```python
from build123d import *

# Parameters (mm, degrees)
CYLINDER014_R     = 1.2
CYLINDER014_DEPTH = 3
CYLINDER013_R     = 0.5
CYLINDER013_DEPTH = 10
ARRAY013_X_COUNT  = 2
ARRAY013_X_PITCH  = 8
ARRAY013_Y_COUNT  = 2
ARRAY013_Y_PITCH  = 8
BOX016_W          = 8
BOX016_H          = 8
BOX016_DEPTH      = 10
TORUS_R           = 0.7
CYLINDER012_R     = 7.7
CYLINDER012_DEPTH = 2.4
CYLINDER003_R     = 10
CYLINDER003_DEPTH = 1.4


with BuildPart() as magnet:
    # Cylinder014 → Cylinder014 (new body)
    with BuildSketch(Plane(origin=(0, -8.5, -1), x_dir=(1, 0, 0), z_dir=(0, 0, 1))):
        Circle(CYLINDER014_R)
    extrude(amount=CYLINDER014_DEPTH)


with BuildPart() as array013:
    # Cylinder013 → Cylinder013 (new body)
    with BuildSketch(Plane(origin=(4, 4, -2), x_dir=(1, 0, 0), z_dir=(0, 0, 1))):
        Circle(CYLINDER013_R)
    extrude(amount=CYLINDER013_DEPTH)

    # Array013 X: Array013 ×2


with BuildPart() as array013_1:
    add(array013.part)
    with Locations(*[(-i * ARRAY013_X_PITCH, 0, 0) for i in range(1, ARRAY013_X_COUNT)]):
        add(array013.part)

    # Array013 Y: Array013 ×2


with BuildPart() as array013_2:
    add(array013_1.part)
    with Locations(*[(0, -i * ARRAY013_Y_PITCH, 0) for i in range(1, ARRAY013_Y_COUNT)]):
        add(array013_1.part)


with BuildPart() as obj1:
    # Box016 → Box016 (new body)
    with BuildSketch(Plane(origin=(-4, -4, -2), x_dir=(1, 0, 0), z_dir=(0, 0, 1))):
        with Locations((4, 4)):
            Rectangle(BOX016_W, BOX016_H)
    extrude(amount=BOX016_DEPTH)


with BuildPart() as torus:
    # Torus → Torus (revolve)
    with BuildSketch(Plane(origin=(0, 0, 1.9), x_dir=(1, 0, 0), z_dir=(0, -1, 0))):
        with Locations((7.7, 0)):
            Circle(TORUS_R)
    revolve(axis=Axis((0, 0, 1.9), (0, 0, 1)))


with BuildPart() as cut017:
    # Cylinder012 → Cylinder012 (new body)
    with BuildSketch(Plane.XY):
        Circle(CYLINDER012_R)
    extrude(amount=CYLINDER012_DEPTH)

    # Cut017: cut Torus
    add(torus.part, mode=Mode.SUBTRACT)


with BuildPart() as magnethalter:
    # Cylinder003 → Cylinder003 (new body)
    with BuildSketch(Plane.XY):
        Circle(CYLINDER003_R)
    extrude(amount=CYLINDER003_DEPTH)

    # Fusion003: union Cut017
    add(cut017.part)

    # Cut018: cut obj1
    add(obj1.part, mode=Mode.SUBTRACT)

    # Cut019: cut Array013
    add(array013_2.part, mode=Mode.SUBTRACT)

    # Cut020: cut Magnet
    add(magnet.part, mode=Mode.SUBTRACT)


solid = magnethalter.part
```
Design review of the part built by this model. Coordinates are the model's own, in mm. A direction names the side the tool comes from. Coordinates: 2 decimals unless noted, no trailing zeros. Order: outer loops, then holes, each group sorted by start corner. A loop starts at its lowest first (then second) coordinate and runs counter-clockwise, first axis right, second up.
1) Wall thickness on line 1 along Z through (x, y) = (4, -8.5); line 2 along Y through (x, z) = (-0.5, 1.3); line 3 along Y through (x, z) = (-2.5, 2): over which ranges is each line inside the solid? List them lowest first.
2) Take a section at A-A, the plane y = 0. Give the boundary of the cut face in (x, z), and give its area (3 significant figures).
3) For faces 4 (the flat face through (0, -4, 1)), 5 (the flat face through (3, -7, 1.4)), 6 (the flat face through (0, -5, 2.4)), list the 3-axis set-ups (+Z, -Z, +X, -X, +Y, -Y) from which the entire face can be reached by the end or side of a thin tool; tool diameter is ignored.
4) Mouldability with a two-part tool opening along X and no side actions: class faces 1 (the flat face through (4.3, 0.1, 0)), 2 (the flat face through (0, 4, 1)), 3 (the cylindrical face through (-2.17, -9.76, 0.69)) as +X half, -X half, draft (parallel to the pull), parting line (faces both ways), or undercut.
5) Take a section at D-D, the plane y = -8.5. Give the boundary of the cut face in (x, z), and give its area (3 significant figures).
6) Take a section at C-C, the plane z = 1.65. Give the boundary of the cut face in (x, y).
7) Take a section at B-B, the plane x = 0. Give the boundary of the cut face in (y, z).
Returned:
1. line 1: z = 0 to 1.4
1. line 2: y = -9.99 to -9.59, -7.41 to -4, 4 to 9.99
1. line 3: y = -6.55 to -4, 4 to 6.55
2. outline: (-10, 0) - (-4, 0) - (-4, 2.4) - (-7.21, 2.4) arc R0.7 cw to (-7.21, 1.4) - (-10, 1.4) - close; (4, 0) - (10, 0) - (10, 1.4) - (7.21, 1.4) arc R0.7 cw to (7.21, 2.4) - (4, 2.4) - close
2. area: 22.9 mm2
3. face 4: +Z, -Z
3. face 5: +Z
3. face 6: +Z, +X, -X, +Y, -Y
4. face 1: draft
4. face 2: undercut
4. face 3: parting line
5. outline: (-5.27, 0) - (-1.2, 0) - (-1.2, 1.4) - (-5.27, 1.4) - close; (1.2, 0) - (5.27, 0) - (5.27, 1.4) - (1.2, 1.4) - close
5. area: 11.4 mm2
6. outline: circle Ø14.09 at (0, 0); hole (-4, -3.5) arc R0.5 ccw (long way) to (-3.5, -4) - (3.5, -4) arc R0.5 ccw (long way) to (4, -3.5) - (4, 3.5) arc R0.5 ccw (long way) to (3.5, 4) - (-3.5, 4) arc R0.5 ccw (long way) to (-4, 3.5) - close
7. outline: (-10, 0) - (-9.7, 0) - (-9.7, 1.4) - (-10, 1.4) - close; (-7.3, 0) - (-4, 0) - (-4, 2.4) - (-7.21, 2.4) arc R0.7 cw to (-7.21, 1.4) - (-7.3, 1.4) - close; (4, 0) - (10, 0) - (10, 1.4) - (7.21, 1.4) arc R0.7 cw to (7.21, 2.4) - (4, 2.4) - close
